Input: part model. Units: mm. Frame: model coordinates. Face numbers are marked on the shaded views. Coordinates: 2 decimals unless noted, no trailing zeros. Write each loop counter-clockwise with the first axis right and the second up, starting at its lowest first coordinate (ties: lowest second). Pieces come first, ordered by that corner, then holes.
from build123d import *

# Parameters (mm, degrees)
SKETCH3_R               = 0.8
CUT_EXTRUDE1_DEPTH      = 2
SKETCH4_R               = 0.8
CUT_EXTRUDE2_DEPTH      = 2
SKETCH6_W               = 0.268563898
SKETCH6_H               = 1.87642035
CUT_EXTRUDE3_DEPTH      = 5
CUT_EXTRUDE3_DEPTH_BACK = 5


with BuildPart() as part:
    # Sketch1 → Revolve1 (revolve)
    with BuildSketch(Plane.XY):
        with BuildLine():
            Line((-3.879111396, 0), (-3.879111396, -12))
            add(Edge.make_bspline(
                [(-3.879111396, -12), (-3.879111396, -12.602750297)],
                knots=[0, 0, 1, 1], degree=1))
            add(Edge.make_bspline(
                [(-3.879111396, -12.602750297), (-4.098454424, -15.2494219), (-0.534839258, -14.725941394), (-0.8, -17.31657115)],
                knots=[0, 0, 0, 0, 1, 1, 1, 1], degree=3))
            Line((-0.8, -17.31657115), (0, -17.31657115))
            Line((0, -17.31657115), (0, 0))
            Line((0, 0), (-3.879111396, 0))
        make_face()
    revolve(axis=Axis((0, 0, 0), (0, -1, 0)))

    # Sketch3 → Cut-Extrude1 (cut)
    with BuildSketch(Plane.XY.offset(3.9)):
        with Locations((0, -1.5)):
            Circle(SKETCH3_R)
    extrude(amount=-CUT_EXTRUDE1_DEPTH, mode=Mode.SUBTRACT)

    # Sketch4 → Cut-Extrude2 (cut)
    with BuildSketch(Plane.XY.offset(-3.9)):
        with Locations((0, -1.5)):
            Circle(SKETCH4_R)
    extrude(amount=CUT_EXTRUDE2_DEPTH, mode=Mode.SUBTRACT)

    # Sketch6 → Cut-Extrude3 (cut, two sides)
    with BuildSketch(Plane(origin=(0, 0, 0), x_dir=(0, 0, -1), z_dir=(1, 0, 0))) as cut_extrude3_sk:
        with Locations((-3.744829447, -1.477966688)):
            Rectangle(SKETCH6_W, SKETCH6_H)
    extrude(amount=CUT_EXTRUDE3_DEPTH, mode=Mode.SUBTRACT)
    extrude(cut_extrude3_sk.sketch, amount=-CUT_EXTRUDE3_DEPTH_BACK, mode=Mode.SUBTRACT)


solid = part.part
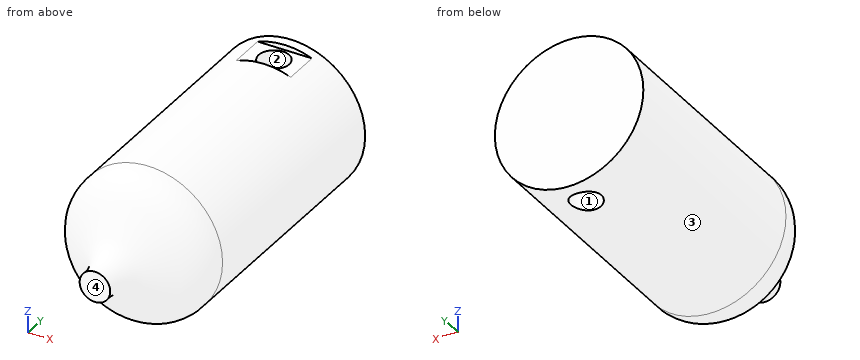
Item 1: Pin query (flat end, axial travel): pin 1 Ø2 at (y, z) = (-5.5, -3) entering from +X; pin 2 Ø1.3 at (x, y) = (0.5, -1.5) entering from +Z; pin 3 Ø1.5 at (x, z) = (-2.5, -2.5) entering from -Y. Return the tip coordinate at first contact, or that it passes through.
Item 2: Pull-direction query (X, two-part tool) for the marked faces 1, 2, 3 and 4; classes: released by +X, released by -X, zero draft, split by the parting line, or undercut.
Item 3: Material intervals for line 1 (Y direction, x = 0, z = -3.2); line 2 (X direction, y = -1.5, z = -2.3); line 3 (X direction, y = -11.25, z = 0), sorted ascending.
Item 4: Section query A-A, the plane y = -1.5. Return loops of the section in (x, z).
The answers:
1. pin 1: stops at x = 3.32
1. pin 2: stops at z = 3.61
1. pin 3: stops at y = -14.68
2. face 1: undercut
2. face 2: undercut
2. face 3: split by the parting line
2. face 4: zero draft
3. line 1: y = -14.35 to -2.3, -0.7 to 0
3. line 2: x = -3.12 to -0.8, 0.8 to 3.12
3. line 3: x = -3.88 to 3.88
4. outline: (-1.42, 3.61) arc R3.88 ccw to (-0.8, -3.8) - (-0.8, -1.9) - (0.8, -1.9) - (0.8, -3.8) arc R3.88 ccw to (1.42, 3.61) - (0.8, 3.61) - (0.8, 1.9) - (-0.8, 1.9) - (-0.8, 3.61) - close
